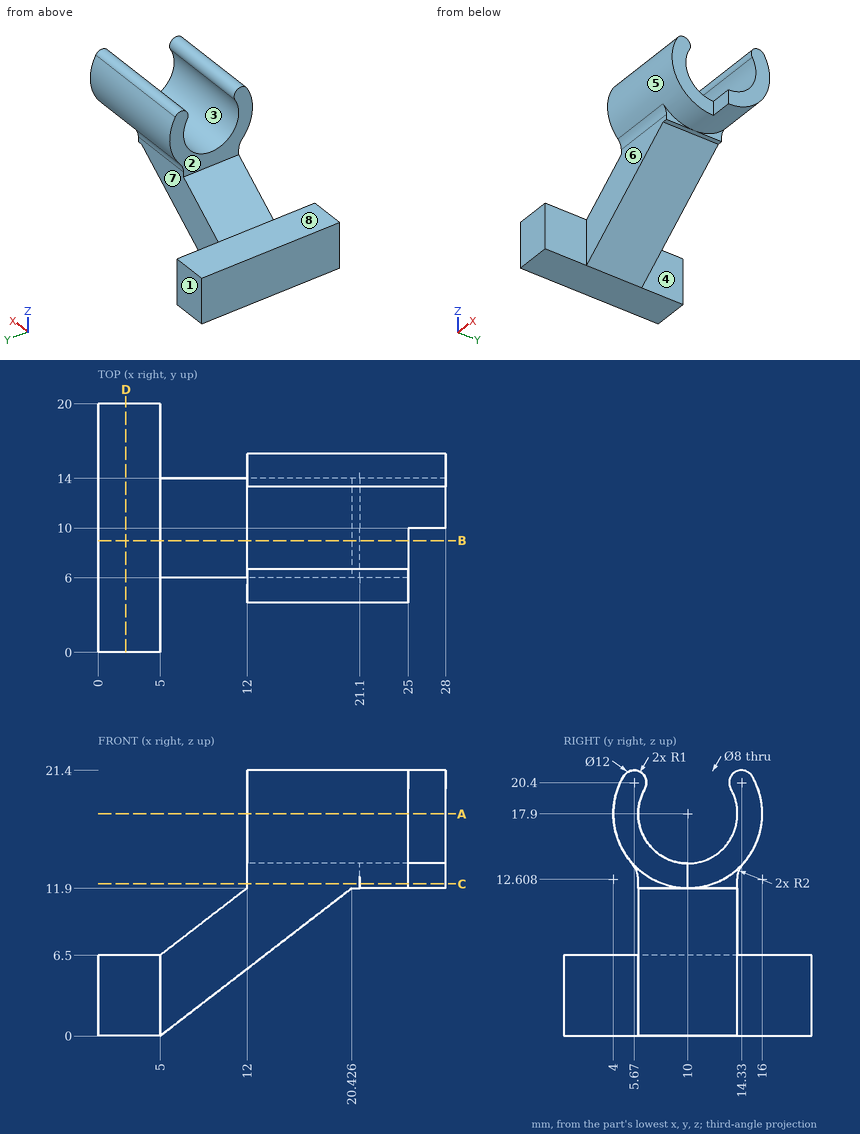
Here's the drawing with two shaded views (mm, measured from the low corner). I have some questions. A direction names the side the tool comes from. Give positions to 0.01 mm unless a question says otherwise; leave off trailing zeros. Loops run counter-clockwise (first coordinate to the right, second up) from the corner with the lowest first, then second, coordinate; pieces in that order, holes last. Notation, with made-up numbers: M -38,1 L -28,1 A12 ccw -28,11 Z; hole C 86,59.5 d5. An arc over 180 degrees is marked long. One line per item, written item: value.
1) Please list where these lines run through material, in increasing order: line 1 (Y direction, x = 22.5, z = 17.9); line 2 (X direction, y = 19, z = 2); line 3 (Z direction, x = 4, y = 16.25).
Geometry check:
line 1: y = 4 to 6, 14 to 16
line 2: x = 0 to 5
line 3: z = 0 to 6.5
2) Imagine slicing it at C-C on z = 12.25. Write out the boundary of the cut face in (x, y).
Geometry check:
outline: M 12,6 L 21.1,6 L 21.1,7.98 L 25,7.98 L 25,10 L 28,10 L 28,12.02 L 21.1,12.02 L 21.1,14 L 12,14 Z
3) On a 3-axis mill with a long thin cutter (end or side, diameter ignored), from which of +Z, -Z, +X, -X, +Y, -Y can I reach the whole of each face in a straight line? I mean the marked faces 4, 5, 6, 7 and 8. Say none if no direction works.
Geometry check:
face 4: +Z, -Z, +X, +Y
face 5: +X
face 6: -Z, +X, -Y
face 7: -Z, +X, +Y
face 8: +Z, -X, +Y, -Y
4) Imagine slicing it at B-B on y = 9. Write out the boundary of the cut face in (x, z).
Geometry check:
outline: M 0,0 L 5,0 L 20.43,11.9 L 21.1,11.9 L 21.1,11.98 L 25,11.98 L 25,14.03 L 12,14.03 L 12,11.9 L 5,6.5 L 0,6.5 Z
5) Thinking about a two-plate mould opening in Y: for the marked faces 1, 2 and 3, which applies, +Y half, -Y half, draft (parallel to the pull), parting line (faces both ways), or undercut?
Geometry check:
face 1: +Y half
face 2: draft
face 3: undercut
6) Imagine slicing it at D-D on x = 2.25. Write out the boundary of the cut face in (y, z), and give its area (3 significant figures).
Geometry check:
outline: M 0,0 L 20,0 L 20,6.5 L 0,6.5 Z
area: 130 mm²
7) Imagine slicing it at A-A on z = 17.9. Write out the boundary of the cut face in (x, y).
Geometry check:
outline: M 12,4 L 25,4 L 25,6 L 12,6 Z; M 12,14 L 28,14 L 28,16 L 12,16 Z
8) I'm going to push flat-ended pins straight in: pin 1 (1 mm diameter, centred on y = 9, z = 13, fed in from +X); pin 2 (3 mm diameter, centred on y = 4, z = 11.5, fed in from -X); pin 3 (0.5 mm diameter, centred on x = 21, y = 10, fed in from -Z); pin 4 (3 mm diameter, centred on y = 18, z = 4, fed in from +X). Where does each tip first touch, or does it pass through?
Geometry check:
pin 1: stops at x = 25
pin 2: passes through
pin 3: stops at z = 11.9
pin 4: stops at x = 5
